Source: CAD feature listing. Evaluate the final solid. Frame: model axes, mm. Face numbers are marked on the shaded views. Round coordinates to 2 decimals unless told otherwise and drop trailing zeros. Write each loop counter-clockwise with the first axis right and the second up, starting at its lowest first coordinate (ties: lowest second). Pieces come first, ordered by that corner, then holes. Notation, with made-up numbers: (73.5, 58) -> (81.5, 58) arc R26 ccw to (81.5, 75) -> close; hole circle Ø8 at (-35.75, 52.25). An arc over 180 degrees is marked (long way). Put each result on its own line as item: value.
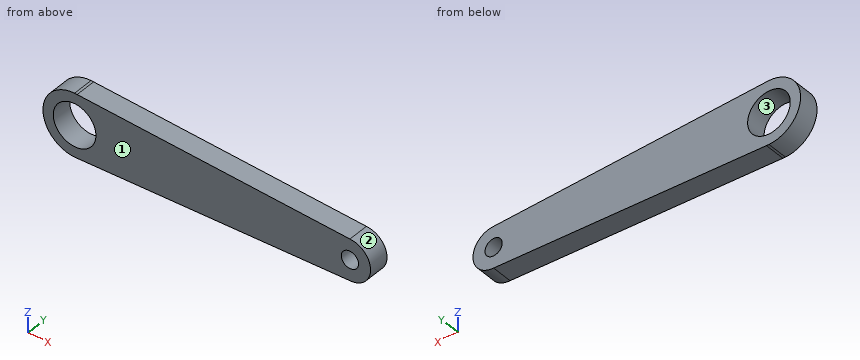
```python
from build123d import *

# Parameters (mm, degrees)
SKETCH1_R           = 3.1
SKETCH1_R_2         = 3
SKETCH1_R_3         = 1.25
BOSS_EXTRUDE1_DEPTH = 3


with BuildPart() as part:
    # Sketch1 → Boss-Extrude1 (new body)
    with BuildSketch(Plane(origin=(0, 0, 0), x_dir=(1, 0, 0), z_dir=(0, 1, 0))):
        with BuildLine():
            Line((40, 3), (0.367412141, 4.585303514))
            ThreePointArc((0.367412141, 4.585303514), (3.380095845, 3.120088473), (4.6, 0))
            ThreePointArc((4.6, 0), (3.380095845, -3.120088473), (0.367412141, -4.585303514))
            Line((0.367412141, -4.585303514), (40, -3))
            ThreePointArc((40, -3), (37, 0), (40, 3))
        make_face()
        with BuildLine():
            Line((0.367412141, 4.585303514), (0, 4.6))
            ThreePointArc((0, 4.6), (-4.6, 0), (0, -4.6))
            Line((0, -4.6), (0.367412141, -4.585303514))
            ThreePointArc((0.367412141, -4.585303514), (3.380095845, -3.120088473), (4.6, 0))
            ThreePointArc((4.6, 0), (3.380095845, 3.120088473), (0.367412141, 4.585303514))
        make_face()
        Circle(SKETCH1_R, mode=Mode.SUBTRACT)
        with Locations((40, 0)):
            Circle(SKETCH1_R_2)
        with Locations((40, 0)):
            Circle(SKETCH1_R_3, mode=Mode.SUBTRACT)
    extrude(amount=BOSS_EXTRUDE1_DEPTH)


solid = part.part
```
Q1. Cut plane B-B on y = 2.1. Output: boundary loops of the cut face in (x, z).
Ans:
outline: (0, -4.6) -> (40, -3) arc R3 ccw to (40, 3) -> (0, 4.6) arc R4.6 ccw to start; hole circle Ø6.2 at (0, 0); hole circle Ø2.5 at (40, 0)
Q2. Cut plane C-C on z = -2. Output: boundary loops of the cut face in (x, y).
Ans:
outline: (-4.14, 0) -> (-2.37, 0) -> (-2.37, 3) -> (-4.14, 3) -> close; (2.37, 0) -> (42.24, 0) -> (42.24, 3) -> (2.37, 3) -> close
Q3. Pin query (flat end, axial travel): pin 1 (1.5 mm diameter, centred on x = 19.5, y = 0.5, fed in from +Z); pin 2 (1 mm diameter, centred on y = 1.5, z = 2.5, fed in from +X). Return the tip coordinate at first contact, or that it passes through.
Ans:
pin 1: stops at z = 3.85
pin 2: stops at x = 42.24
Q4. Material intervals for line 1 (X direction, y = 2.1, z = 0); line 2 (Z direction, x = 40, y = 1.55); line 3 (X direction, y = 2.3, z = -2.5), sorted ascending. Write a range as [from, to].
Ans:
line 1: x = [-4.6, -3.1], [3.1, 38.75], [41.25, 43]
line 2: z = [-3, -1.25], [1.25, 3]
line 3: x = [-3.86, -1.83], [1.83, 41.66]
Q5. Draft query along Z for the marked faces 1, 2 and 3. Return one class per face: +Z half, -Z half, draft (parallel to the pull), parting line (faces both ways), or undercut.
Ans:
face 1: draft
face 2: parting line
face 3: undercut
Q6. Cut plane D-D on x = 15. Output: boundary loops of the cut face in (y, z), and give its area (3 significant figures).
Ans:
outline: (0, -4) -> (3, -4) -> (3, 4) -> (0, 4) -> close
area: 24.0 mm^2
Q7. Cut plane A-A on z = 0. Output: boundary loops of the cut face in (x, y), and give its area (3 significant figures).
Ans:
outline: (-4.6, 0) -> (-3.1, 0) -> (-3.1, 3) -> (-4.6, 3) -> close; (3.1, 0) -> (38.75, 0) -> (38.75, 3) -> (3.1, 3) -> close; (41.25, 0) -> (43, 0) -> (43, 3) -> (41.25, 3) -> close
area: 117 mm^2
